Verification items for the finished model (mm, model axes). Give positions to 0.01 mm unless a question says otherwise; leave off trailing zeros. Loops run counter-clockwise (first coordinate to the right, second up) from the corner with the lowest first, then second, coordinate; pieces in that order, holes last. Notation, with made-up numbers: (1.25, 51.5) - (9.25, 51.5) arc R21 cw to (9.25, 81.5) - close; hole circle Ø10 at (78.25, 58). An arc over 180 degrees is marked (long way). One line per item, written item: value. Start each with the question number.
1. Sectioned sample at A-A (z = 13.5). Record the cut outline in (x, y), plus the area to 3 significant figures.
2. Sectioned sample at B-B (x = -31.5). Record the cut outline in (y, z), plus the area to 3 significant figures.
3. Gauge pin test, flat ends, axial feed: pin 1 (4 mm diameter, centred on x = -19.5, z = 21, fed in from +Y); pin 2 (0.6 mm diameter, centred on x = -33.5, y = 26, fed in from -Z); pin 3 (1 mm diameter, centred on x = -20.5, z = 11.5, fed in from -Y). Record the tip position at first contact, or that the pin passes through.
4. Sectioned sample at D-D (x = -22). Record the cut outline in (y, z).
5. Sectioned sample at C-C (y = 28.3). Record the cut outline in (x, z), plus the area to 3 significant figures.
6. Scan lines: L1, parallel to Y at x = -30, z = 11; L2, parallel to Z at x = -33.5, y = 26.1; L3, parallel to Y at x = -38, z = 14.5. Record each from-to range of solid material in increasing order. Write a range as [from, to].
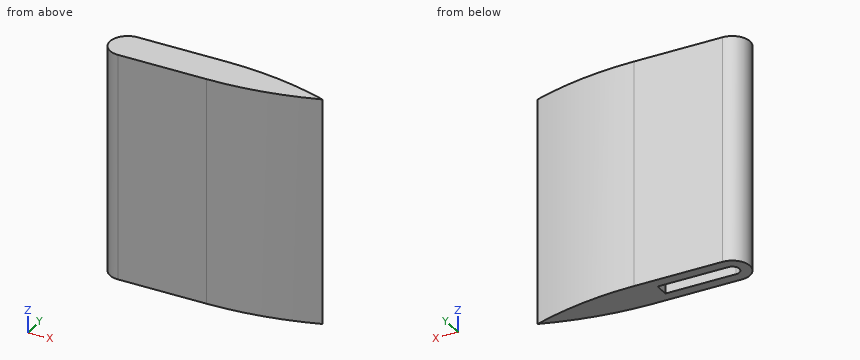
from build123d import *

# Parameters (mm, degrees)
BOSS_EXTRU_1_DEPTH      = 32
ENL_V_MAT_EXTRU_2_DEPTH = 25


with BuildPart() as part:
    # Esquisse1 → Boss.-Extru.1 (new body)
    with BuildSketch(Plane.XY):
        with BuildLine():
            Line((-37.240452994, 28.735655929), (-24.740452994, 28.735655929))
            ThreePointArc((-24.740452994, 28.735655929), (-17.136999831, 28.106374906), (-9.740452994, 26.235655929))
            ThreePointArc((-9.740452994, 26.235655929), (-17.136999831, 24.364936952), (-24.740452994, 23.735655929))
            Line((-24.740452994, 23.735655929), (-37.240452994, 23.735655929))
            ThreePointArc((-37.240452994, 23.735655929), (-39.740452994, 26.235655929), (-37.240452994, 28.735655929))
        make_face()
    extrude(amount=BOSS_EXTRU_1_DEPTH)

    # Esquisse3 → Enlèv. mat.-Extru.2 (cut)
    with BuildSketch(Plane(origin=(0, 0, 0), x_dir=(-1, 0, 0), z_dir=(0, 0, -1))):
        with BuildLine():
            Line((37.240452994, 25.235655929), (27.240452994, 25.235655929))
            Line((27.240452994, 25.235655929), (27.240452994, 27.235655929))
            Line((27.240452994, 27.235655929), (37.240452994, 27.235655929))
            ThreePointArc((37.240452994, 27.235655929), (38.240452994, 26.235655929), (37.240452994, 25.235655929))
        make_face()
    extrude(amount=-ENL_V_MAT_EXTRU_2_DEPTH, mode=Mode.SUBTRACT)


solid = part.part
Results are:
1. outline: (-37.24, 23.74) - (-24.74, 23.74) arc R46.25 ccw to (-9.74, 26.24) arc R46.25 ccw to (-24.74, 28.74) - (-37.24, 28.74) arc R2.5 ccw to start; hole (-37.24, 25.24) - (-27.24, 25.24) - (-27.24, 27.24) - (-37.24, 27.24) arc R1 ccw to start
1. area: 101 mm^2
2. outline: (23.74, 0) - (25.24, 0) - (25.24, 25) - (27.24, 25) - (27.24, 0) - (28.74, 0) - (28.74, 32) - (23.74, 32) - close
2. area: 110 mm^2
3. pin 1: stops at y = 28.62
3. pin 2: stops at z = 25
3. pin 3: stops at y = 23.89
4. outline: (23.82, 0) - (28.65, 0) - (28.65, 32) - (23.82, 32) - close
5. outline: (-38.65, 0) - (-18.41, 0) - (-18.41, 32) - (-38.65, 32) - close
5. area: 648 mm^2
6. L1: y = [23.74, 25.24], [27.24, 28.74]
6. L2: z = [25, 32]
6. L3: y = [23.85, 25.59], [26.89, 28.62]
